```python
from build123d import *

# Parameters (mm, degrees)
F0_R     = 1.6
F1_DEPTH = 1


# Not quite as in the source:
# - ends of sketch curves that miss each other by under 0.0002 mm in the source are joined


with BuildPart() as f1:
    # F0 (on Top) → F1 (new body)
    with BuildSketch(Plane.XY):
        Polygon((102.2, 56.7), (113.5, 56.7), (118.8, 56.7), (118.8, 69), (-118.8, 69), (-118.8, -69), (118.8, -69), (118.8, 19.1), (118.7999, 19.1001), (113.553, 19.1001), (104.2105, 19.1005), (104.2, -22.45), (88.8825, -22.45), (77.8, -22.45), (77.8, -11.8), (57.15, -11.8), (57.15, 5.75), (62.2, 5.75), (62.2, 12.6), (37.3752, 12.5999), (-30.4, 12.6), (-30.4, 64), (37.3639, 64), (61.18, 64), (78.995, 64), (79.01, 64), (79.0100016935, 63.9849983065), (79.012, 46.283), (88.0852, 46.283), (102.2, 46.282), align=None)
        with Locations((-115.8, -66)):
            Circle(F0_R, mode=Mode.SUBTRACT)
        with Locations((-75.3, -66)):
            Circle(F0_R, mode=Mode.SUBTRACT)
        with Locations((-96.002, -45.2007)):
            Circle(F0_R, mode=Mode.SUBTRACT)
        with Locations((-37.3, -66)):
            Circle(F0_R, mode=Mode.SUBTRACT)
        with Locations((-40.7, -50.30003)):
            Circle(F0_R, mode=Mode.SUBTRACT)
        with Locations((-115.8, -12.8)):
            Circle(F0_R, mode=Mode.SUBTRACT)
        with Locations((-99.4, -11.9)):
            Circle(F0_R, mode=Mode.SUBTRACT)
        with Locations((-87.9916, -11.4944)):
            Circle(F0_R, mode=Mode.SUBTRACT)
        with Locations((-62.3953, -11.5044)):
            Circle(F0_R, mode=Mode.SUBTRACT)
        with Locations((-35.9953, -11.5044)):
            Circle(F0_R, mode=Mode.SUBTRACT)
        with Locations((0.5, -66)):
            Circle(F0_R, mode=Mode.SUBTRACT)
        with Locations((38.7, -66)):
            Circle(F0_R, mode=Mode.SUBTRACT)
        with Locations((38.6047, -38.8044)):
            Circle(F0_R, mode=Mode.SUBTRACT)
        with Locations((59.7, -66)):
            Circle(F0_R, mode=Mode.SUBTRACT)
        with Locations((88.4, -66)):
            Circle(F0_R, mode=Mode.SUBTRACT)
        with Locations((116.2, -66)):
            Circle(F0_R, mode=Mode.SUBTRACT)
        with Locations((59.6946, -37.8013)):
            Circle(F0_R, mode=Mode.SUBTRACT)
        with Locations((116.2, -39.2)):
            Circle(F0_R, mode=Mode.SUBTRACT)
        with Locations((18.7, -28.7)):
            Circle(F0_R, mode=Mode.SUBTRACT)
        with Locations((18.7, -7.2)):
            Circle(F0_R, mode=Mode.SUBTRACT)
        with Locations((38.6, -15.9)):
            Circle(F0_R, mode=Mode.SUBTRACT)
        with Locations((54.3, -11.30003)):
            Circle(F0_R, mode=Mode.SUBTRACT)
        with Locations((38.5947, -0.0044)):
            Circle(F0_R, mode=Mode.SUBTRACT)
        with Locations((91, -31.2)):
            Circle(F0_R, mode=Mode.SUBTRACT)
        with Locations((59.7, -14.6)):
            Circle(F0_R, mode=Mode.SUBTRACT)
        with Locations((71.6, -16.3)):
            Circle(F0_R, mode=Mode.SUBTRACT)
        with Locations((116.2, -11.2)):
            Circle(F0_R, mode=Mode.SUBTRACT)
        with Locations((-99.392, 11.7993)):
            Circle(F0_R, mode=Mode.SUBTRACT)
        with Locations((-74.0947, 5.3044)):
            Circle(F0_R, mode=Mode.SUBTRACT)
        with Locations((-85.3, 15.3)):
            Circle(F0_R, mode=Mode.SUBTRACT)
        with Locations((-115.8, 20.5)):
            Circle(F0_R, mode=Mode.SUBTRACT)
        with Locations((-66.6053, 21.28557)):
            Circle(F0_R, mode=Mode.SUBTRACT)
        with Locations((-75.0953, 28.4956)):
            Circle(F0_R, mode=Mode.SUBTRACT)
        with Locations((-35.9953, 6.4956)):
            Circle(F0_R, mode=Mode.SUBTRACT)
        with Locations((-55.2953, 15.3056)):
            Circle(F0_R, mode=Mode.SUBTRACT)
        with Locations((-39.5853, 21.8056)):
            Circle(F0_R, mode=Mode.SUBTRACT)
        with Locations((-47.8, 31.4)):
            Circle(F0_R, mode=Mode.SUBTRACT)
        with Locations((-32.8, 30.8)):
            Circle(F0_R, mode=Mode.SUBTRACT)
        with Locations((-99.392, 35.3993)):
            Circle(F0_R, mode=Mode.SUBTRACT)
        with BuildLine():
            ThreePointArc((-71.6712000014, 25.5657995631), (-72.0236133171, 25.7129538657), (-72.1690001854, 26.0661000003))
            Line((-72.1690001854, 26.0661000003), (-72.169, 30.6661))
            ThreePointArc((-72.169, 30.6661), (-72.022760123, 31.017660123), (-71.6711999992, 31.1638997499))
            Line((-71.6711999992, 31.1638997499), (-71.6712, 44.6361))
            ThreePointArc((-71.6712, 44.6361), (-72.022760123, 44.782339877), (-72.1689997499, 45.1339000008))
            Line((-72.1689997499, 45.1339000008), (-72.169, 49.7339))
            ThreePointArc((-72.169, 49.7339), (-72.0236133171, 50.0870461343), (-71.6712000014, 50.2342004369))
            Line((-71.6712000014, 50.2342004369), (-62.6288, 50.2342))
            ThreePointArc((-62.6288, 50.2342), (-62.2763866829, 50.0870461343), (-62.1309998146, 49.7338999997))
            Line((-62.1309998146, 49.7338999997), (-62.131, 45.1339))
            ThreePointArc((-62.131, 45.1339), (-62.277239877, 44.782339877), (-62.6288000008, 44.6361002501))
            Line((-62.6288000008, 44.6361002501), (-62.6288, 31.1639))
            ThreePointArc((-62.6288, 31.1639), (-62.277239877, 31.017660123), (-62.1310002501, 30.6660999992))
            Line((-62.1310002501, 30.6660999992), (-62.131, 26.0661))
            ThreePointArc((-62.131, 26.0661), (-62.2763866829, 25.7129538657), (-62.6287999986, 25.5657995631))
            Line((-62.6287999986, 25.5657995631), (-71.6712000014, 25.5657995631))
        make_face(mode=Mode.SUBTRACT)
        with Locations((-75.0953, 47.9056)):
            Circle(F0_R, mode=Mode.SUBTRACT)
        with Locations((-115.8, 66)):
            Circle(F0_R, mode=Mode.SUBTRACT)
        with Locations((-98.1, 65.4)):
            Circle(F0_R, mode=Mode.SUBTRACT)
        with Locations((-84.8, 66)):
            Circle(F0_R, mode=Mode.SUBTRACT)
        with Locations((-63.3, 66)):
            Circle(F0_R, mode=Mode.SUBTRACT)
        with Locations((-47.7953, 44.6956)):
            Circle(F0_R, mode=Mode.SUBTRACT)
        with Locations((-32.8, 45.1)):
            Circle(F0_R, mode=Mode.SUBTRACT)
        with Locations((-33.3, 66)):
            Circle(F0_R, mode=Mode.SUBTRACT)
        with Locations((-3.3, 66)):
            Circle(F0_R, mode=Mode.SUBTRACT)
        with Locations((18.7, 10)):
            Circle(F0_R, mode=Mode.SUBTRACT)
        with Locations((48.3948, 10.0954)):
            Circle(F0_R, mode=Mode.SUBTRACT)
        with Locations((59.698, 8.2993)):
            Circle(F0_R, mode=Mode.SUBTRACT)
        with Locations((116.2, 16.8)):
            Circle(F0_R, mode=Mode.SUBTRACT)
        with BuildLine():
            ThreePointArc((26.5840005, 64.4042105039), (24.868001, 66), (26.5840005, 67.5957894961))
            ThreePointArc((26.5840005, 67.5957894961), (27.7895872613, 67.1716653106), (28.3, 66))
            ThreePointArc((28.3, 66), (27.7895872613, 64.8283346894), (26.5840005, 64.4042105039))
        make_face(mode=Mode.SUBTRACT)
        with Locations((56.7, 66)):
            Circle(F0_R, mode=Mode.SUBTRACT)
        with Locations((86.7, 52.5)):
            Circle(F0_R, mode=Mode.SUBTRACT)
        with Locations((86.7, 66)):
            Circle(F0_R, mode=Mode.SUBTRACT)
        with Locations((116.2, 66)):
            Circle(F0_R, mode=Mode.SUBTRACT)
    extrude(amount=F1_DEPTH)


solid = f1.part
```
Verification items for the finished model (mm, model axes). Round coordinates to 2 decimals unless told otherwise and drop trailing zeros. Write each loop counter-clockwise with the first axis right and the second up, starting at its lowest first coordinate (ties: lowest second). Pieces come first, ordered by that corner, then holes. Notation, with made-up numbers: (41.25, 39) -> (62.25, 39) arc R20 cw to (62.25, 61) -> close; hole circle Ø8 at (8.25, 85). An arc over 180 degrees is marked (long way). Write each question's results on one line, items separated by ' | '.
Q1. Thickness scan on probe 1 along X at (y, z) = (12, 0.1); probe 2 along Y at (x, z) = (-71, 0.9); probe 3 along X at (y, z) = (50.5, 0.7). Record the ranges inside material, lowest first.
Derived:
probe 1: x = -118.8 to -100.98, -97.8 to 62.2, 104.21 to 118.8 | probe 2: y = -69 to 25.57, 50.23 to 69 | probe 3: x = -118.8 to -30.4, 79.01 to 102.2
Q2. Sectioned sample at B-B, the plane x = 98. Record the boundary of the cut face in (y, z).
Derived:
outline: (-69, 0) -> (-22.45, 0) -> (-22.45, 1) -> (-69, 1) -> close; (46.28, 0) -> (69, 0) -> (69, 1) -> (46.28, 1) -> close
Q3. Sectioned sample at A-A, the plane x = -8. Record the boundary of the cut face in (y, z).
Derived:
outline: (-69, 0) -> (12.6, 0) -> (12.6, 1) -> (-69, 1) -> close; (64, 0) -> (69, 0) -> (69, 1) -> (64, 1) -> close
Q4. Sectioned sample at C-C, the plane z = 0.8. Give the number of separate pieces and of enclosed holes in the cut face, and give its area (3 significant figures).
Derived:
separate pieces: 1 | enclosed holes: 58 | area: 23,700 mm²
